```python
from build123d import *

# Parameters (mm, degrees)
SKETCH1_W           = 19.05
SKETCH1_H           = 29.845
BOSS_EXTRUDE1_DEPTH = 11.43
SKETCH2_R           = 2.54
CUT_EXTRUDE1_DEPTH  = 11.43
SKETCH3_W           = 19.05
SKETCH3_H           = 7.62
CUT_EXTRUDE2_DEPTH  = 1.27


with BuildPart() as part:
    # Sketch1 → Boss-Extrude1 (new body)
    with BuildSketch(Plane.XY):
        with Locations((1.663095238, -4.906130952)):
            Rectangle(SKETCH1_W, SKETCH1_H)
    extrude(amount=BOSS_EXTRUDE1_DEPTH)

    # Sketch2 → Cut-Extrude1 (cut)
    with BuildSketch(Plane.XY.offset(11.43)):
        with Locations((1.663095238, 7.730369048)):
            Circle(SKETCH2_R)
        with Locations((1.663095238, -17.669630952)):
            Circle(SKETCH2_R)
    extrude(amount=-CUT_EXTRUDE1_DEPTH, mode=Mode.SUBTRACT)

    # Sketch3 → Cut-Extrude2 (cut)
    with BuildSketch(Plane.XY.offset(11.43)):
        with Locations((1.663095238, 6.206369048)):
            Rectangle(SKETCH3_W, SKETCH3_H)
        with Locations((1.663095238, -16.018630952)):
            Rectangle(SKETCH3_W, SKETCH3_H)
    extrude(amount=-CUT_EXTRUDE2_DEPTH, mode=Mode.SUBTRACT)


solid = part.part
```
Here's how the part is built. I have some questions about the finished solid (model axes, mm). A direction names the side the tool comes from. Coordinates: 2 decimals unless noted, no trailing zeros. Loops run counter-clockwise (first coordinate to the right, second up) from the corner with the lowest first, then second, coordinate; pieces in that order, holes last. Notation, with made-up numbers: (6.5, -25) - (25.5, -25) arc R21 cw to (25.5, -15) - close; hole circle Ø8 at (-39, -21.5). An arc over 180 degrees is marked (long way). Return JSON: item names as keys, results as strings. Group by question number.
Item 1: Will these pins go through, and if not, where does the flat tip stop? P1, Ø4.5, axis at x = 1.66, y = -17.67, coming from the -Z side; P2, Ø1.4, axis at x = 0, z = 11, coming from the +Y side; P3, Ø3, axis at x = -4.5, y = -16, coming from the +Z side.
Item 2: I need wall thicknesses on line 1 (Y direction, x = 4, z = 2); line 2 (Z direction, x = -5.25, y = 6.5); line 3 (Y direction, x = -5.5, z = 10.5). Which ranges of each line are inside material? Lowest first, please. Write a range as from..to.
Item 3: If we section it at A-A on z = 5: Write out the boundary of the cut face in (x, y), and give its area (3 significant figures).
Item 4: If we section it at C-C on y = -12.75: Write out the boundary of the cut face in (x, z).
Item 5: If we section it at B-B on x = -1.75: Write out the boundary of the cut face in (y, z), and give its area (3 significant figures).
Item 6: On a 3-axis mill with a long thin cutter (end or side, diameter ignored), from which of +Z, -Z, +X, -X, +Y, -Y can I reach the whole of each face in a straight line? I mean faces 5 (the face through (2, 5, 10.16)), 6 (the face through (-4, 10.016, 5)), 7 (the face through (2, -15, 10.16)). Say none if no direction works.
Item 7: We'd pull the mould along Y, two halves only. Please class faces 1 (the face through (2, 2.396, 11)), 2 (the face through (2, -5, 0)), 3 (the face through (1.567, 5.192, 5.151)), 4 (the face through (1.76, -15.13, 5.15)): +Y half, -Y half, draft (parallel to the pull), parting line (faces both ways), or undercut.
Calculated:
{
 "1": {"P1": "passes through", "P2": "stops at y = 2.4", "P3": "stops at z = 10.16"},
 "2": {"line 1": "y = -19.83..-18.66, -16.67..6.74, 8.73..10.02", "line 2": "z = 0..10.16", "line 3": "y = -12.21..2.4"},
 "3": {"outline": "(-7.86, -19.83) - (0.33, -19.83) arc R2.54 cw (long way) to (3, -19.83) - (11.19, -19.83) - (11.19, 10.02) - (2.77, 10.02) arc R2.54 cw (long way) to (0.56, 10.02) - (-7.86, 10.02) - close", "area": "529 mm^2"},
 "4": {"outline": "(-7.86, 0) - (11.19, 0) - (11.19, 10.16) - (-7.86, 10.16) - close"},
 "5": {"outline": "(-19.83, 0) - (10.02, 0) - (10.02, 10.16) - (2.4, 10.16) - (2.4, 11.43) - (-12.21, 11.43) - (-12.21, 10.16) - (-19.83, 10.16) - close", "area": "322 mm^2"},
 "6": {"face 5": "+Z, +X, -X, +Y", "face 6": "+Z, -Z, +X, -X, +Y", "face 7": "+Z, +X, -X, -Y"},
 "7": {"face 1": "+Y half", "face 2": "draft", "face 3": "undercut", "face 4": "undercut"}
}
